Read the model definition and answer for the solid it produces. Units are mm, in the model's axes. A direction names the side the tool comes from. Round coordinates to 2 decimals unless told otherwise and drop trailing zeros. Order: outer loops, then holes, each group sorted by start corner. A loop starts at its lowest first (then second) coordinate and runs counter-clockwise, first axis right, second up. Notation, with made-up numbers: (54.25, 4.25) - (79.25, 4.25) arc R17 cw to (79.25, 16.25) - close; hole circle Ø5 at (-27, -18.5). An arc over 180 degrees is marked (long way). Put each result on its own line as item: value. Start each with the question number.
Q1. Section D-D on y = 28 is taken. Give the vertices of the cut face in (x, z).
Q2. Section A-A on z = 0 is taken. Give the vertices of the cut face in (x, y) (3 decimals), then the cut area to 3 significant figures.
Q3. Section C-C on z = -7 is taken. Give the vertices of the cut face in (x, y), then the cut area to 3 significant figures.
Q4. Find the intervals of material crossed by line 1 along Z through (x, y) = (0, 9.95); line 2 along Z through (x, y) = (0, 12.5), in increasing order. Write a range as from..to.
Q5. For a pull along Y with two mould halves and no side action, classify faces 4 (the face through (-6, 14, 0)), 5 (the face through (-0.37, 45.94, 0.07)), 6 (the face through (0, 12.017, 0)) as pulls with the +Y half, pulls with the -Y half, needs draft (parallel to the pull), parting line crosses it, or undercut.
Q6. Which of the six approach directions +Z, -Z, +X, -X, +Y, -Y give full straight-line access (tool end or side, diameter ignored) to faces 1 (the face through (4.482, 37.833, -1.411)), 2 (the face through (-0.74, 10.41, 3.35)), 3 (the face through (-1.323, 13.875, -10.074))?
Q7. Each of these flat-tipped pins is pushed along its axis until it touches: pin 1 Ø2 at (y, z) = (32, 0.5) entering from +X; pin 2 Ø5.5 at (x, z) = (0, -1) entering from -Y; pin 3 Ø10 at (x, y) = (0, 33.5) entering from +Z; pin 4 Ø4 at (x, z) = (0, 0) entering from -Y. Where does it stop, or does it pass through?
Q8. Section B-B on x = 0 is taken. Give the vertices of the cut face in (y, z).
from build123d import *

# Parameters (mm, degrees)
SKETCH1_R               = 10.16
SKETCH1_R_2             = 1.000000032
BOSS_EXTRUDE1_DEPTH     = 19.05
SKETCH2_R               = 4.699
BOSS_EXTRUDE2_DEPTH     = 38.1
SKETCH4_R               = 10.16
CUT_EXTRUDE2_DEPTH      = 8.842000096
CUT_EXTRUDE3_START      = 8.842
SKETCH3_R               = 3.429
CUT_EXTRUDE3_DEPTH      = 3.175
SKETCH5_R               = 1.726999975
CUT_EXTRUDE4_DEPTH      = 11.16
CUT_EXTRUDE4_DEPTH_BACK = 11.16


with BuildPart() as part:
    # Sketch1 → Boss-Extrude1 (new body)
    with BuildSketch(Plane(origin=(0, 0, 0), x_dir=(1, 0, 0), z_dir=(0, 1, 0))):
        Circle(SKETCH1_R)
        with Locations((6.99999997, 0)):
            Circle(SKETCH1_R_2, mode=Mode.SUBTRACT)
        with Locations((0, -6.99999997)):
            Circle(SKETCH1_R_2, mode=Mode.SUBTRACT)
        with Locations((-6.99999997, 0)):
            Circle(SKETCH1_R_2, mode=Mode.SUBTRACT)
        with Locations((0, 6.99999997)):
            Circle(SKETCH1_R_2, mode=Mode.SUBTRACT)
    extrude(amount=BOSS_EXTRUDE1_DEPTH)

    # Sketch2 → Boss-Extrude2 (add)
    with BuildSketch(Plane(origin=(0, 19.05, 0), x_dir=(1, 0, 0), z_dir=(0, 1, 0))):
        Circle(SKETCH2_R)
    extrude(amount=BOSS_EXTRUDE2_DEPTH)

    # Sketch4 → Cut-Extrude2 (cut)
    with BuildSketch(Plane.XZ):
        Circle(SKETCH4_R)
    extrude(amount=-CUT_EXTRUDE2_DEPTH, mode=Mode.SUBTRACT)

    # Sketch3 → Cut-Extrude3 (cut)
    with BuildSketch(Plane(origin=(0, 0, 0), x_dir=(1, 0, 0), z_dir=(0, 1, 0)).offset(CUT_EXTRUDE3_START)):
        Circle(SKETCH3_R)
    extrude(amount=CUT_EXTRUDE3_DEPTH, mode=Mode.SUBTRACT)

    # Sketch5 → Cut-Extrude4 (cut, two sides)
    with BuildSketch(Plane.XY) as cut_extrude4_sk:
        with Locations((0, 47.625)):
            Circle(SKETCH5_R)
    extrude(amount=CUT_EXTRUDE4_DEPTH, mode=Mode.SUBTRACT)
    extrude(cut_extrude4_sk.sketch, amount=-CUT_EXTRUDE4_DEPTH_BACK, mode=Mode.SUBTRACT)


solid = part.part
Findings:
1. outline: circle Ø9.4 at (0, 0)
2. outline: (-10.16, 8.842) - (-8, 8.842) - (-8, 19.05) - (-10.16, 19.05) - close; (-6, 8.842) - (-3.429, 8.842) - (-3.429, 12.017) - (3.429, 12.017) - (3.429, 8.842) - (6, 8.842) - (6, 19.05) - (4.699, 19.05) - (4.699, 57.15) - (-4.699, 57.15) - (-4.699, 19.05) - (-6, 19.05) - close; (8, 8.842) - (10.16, 8.842) - (10.16, 19.05) - (8, 19.05) - close; hole circle Ø3.454 at (0, 47.625)
2. area: 494 mm2
3. outline: (-7.36, 8.84) - (-1, 8.84) - (-1, 19.05) - (-7.36, 19.05) - close; (1, 8.84) - (7.36, 8.84) - (7.36, 19.05) - (1, 19.05) - close
3. area: 130 mm2
4. line 1: -10.16..-8, -6..-3.43, 3.43..6, 8..10.16
4. line 2: -10.16..-8, -6..6, 8..10.16
5. face 4: needs draft
5. face 5: undercut
5. face 6: pulls with the -Y half
6. face 1: +Y
6. face 2: -Y
6. face 3: +Y, -Y
7. pin 1: x = 4.7
7. pin 2: y = 8.84
7. pin 3: z = 4.7
7. pin 4: y = 12.02
8. outline: (8.84, -10.16) - (19.05, -10.16) - (19.05, -8) - (8.84, -8) - close; (8.84, -6) - (19.05, -6) - (19.05, -4.7) - (45.9, -4.7) - (45.9, 4.7) - (19.05, 4.7) - (19.05, 6) - (8.84, 6) - (8.84, 3.43) - (12.02, 3.43) - (12.02, -3.43) - (8.84, -3.43) - close; (8.84, 8) - (19.05, 8) - (19.05, 10.16) - (8.84, 10.16) - close; (49.35, -4.7) - (57.15, -4.7) - (57.15, 4.7) - (49.35, 4.7) - close
